from build123d import *

# Parameters (mm, degrees)
SKETCH133_W       = 5
SKETCH133_H       = 20
PAD080_DEPTH      = 20
SKETCH134_W       = 2.5
SKETCH134_H       = 15.6
POCKET028_DEPTH   = 18
CYLINDER086_R     = 6.5
CYLINDER086_DEPTH = 3
PAD081_DEPTH      = 2.5


with BuildPart() as part:
    # Sketch133 → Pad080 (new body)
    with BuildSketch(Plane.XY):
        with Locations((2.5, 0)):
            Rectangle(SKETCH133_W, SKETCH133_H)
    extrude(amount=-PAD080_DEPTH)

    # Sketch134 → Pocket028 (cut)
    with BuildSketch(Plane(origin=(2.5, 0, 0), x_dir=(1, 0, 0), z_dir=(0, 0, 1))):
        Rectangle(SKETCH134_W, SKETCH134_H)
    extrude(amount=-POCKET028_DEPTH, mode=Mode.SUBTRACT)

    # Cylinder086 → Cylinder086 (cut)
    with BuildSketch(Plane(origin=(3, 0, -11), x_dir=(0, 1, 0), z_dir=(1, 0, 0))):
        Circle(CYLINDER086_R)
    extrude(amount=CYLINDER086_DEPTH, mode=Mode.SUBTRACT)

    # Sketch135 → Pad081 (join, symmetric)
    with BuildSketch(Plane(origin=(0, 0, -2), x_dir=(1, 0, 0), z_dir=(0, -1, 0))):
        Polygon((-8, 0), (0, 0), (0, -16), align=None)
    extrude(amount=PAD081_DEPTH, both=True)


with BuildPart() as part_1:
    # Body118 placement: moved
    add(part.part.moved(Location((5, 0, 0))))


solid = part_1.part
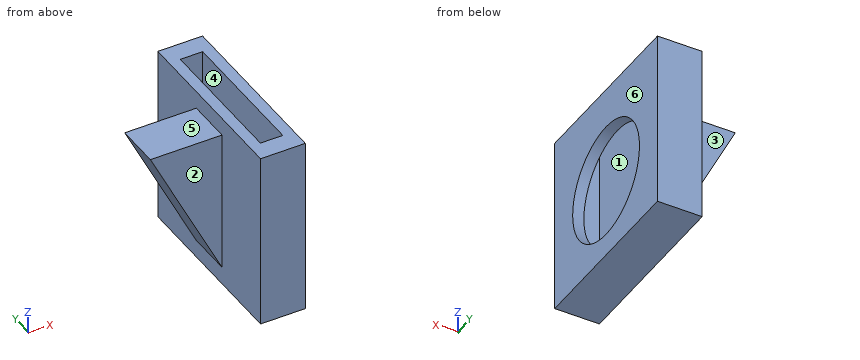
Can you work these out from the model? Positions are in its coordinate system, mm. Face numbers are marked on the shaded views. A direction names the side the tool comes from. Give positions to 0.01 mm unless a question says otherwise; leave off trailing zeros. Order: outer loops, then holes, each group sorted by start corner. A loop starts at its lowest first (then second) coordinate and runs counter-clockwise, first axis right, second up. Notation, with made-up numbers: M 19,66 L 61,66 A18 cw 61,84 Z; hole C -17.5,74.25 d8. An arc over 180 degrees is marked long. One line per question, with ' | ' between items.
Item 1: We'd pull the mould along X, two halves only. Please class the marked faces 4, 5 and 6: released by +X, released by -X, zero draft, split by the parting line, or undercut.
Answer block:
face 4: undercut | face 5: zero draft | face 6: released by +X
Item 2: Please list where these lines run through material, in increasing order: L1, parallel to Z at x = 9.1, y = 0; L2, parallel to X at y = -4, z = -1.5; L3, parallel to Y at x = 8, z = -6.25.
Answer block:
L1: z = -20 to -17.5, -4.5 to 0 | L2: x = 5 to 6.25, 8.75 to 10 | L3: y = -10 to -7.8, 7.8 to 10
Item 3: Suppose I cut it at C-C, the plane x = 9.25. Write out the boundary of the cut face in (y, z).
Answer block:
outline: M -10,-20 L 10,-20 L 10,0 L -10,0 Z; hole C 0,-11 d13
Item 4: Suppose I cut it at B-B, the plane z = -17. Write out the boundary of the cut face in (x, y).
Answer block:
outline: M 4.5,-2.5 L 5,-2.5 L 5,-10 L 10,-10 L 10,-2.5 L 8.75,-2.5 L 8.75,-7.8 L 6.25,-7.8 L 6.25,7.8 L 8.75,7.8 L 8.75,2.5 L 10,2.5 L 10,10 L 5,10 L 5,2.5 L 4.5,2.5 Z
Item 5: I'm going to push flat-ended pins straight in: pin 1 Ø4 at (x, y) = (0.5, 2) entering from -Z; pin 2 Ø6 at (y, z) = (4, -13) entering from -X; pin 3 Ø4 at (y, z) = (-0.5, -14.5) entering from -X. Where does each tip first touch, or does it pass through?
Answer block:
pin 1: stops at z = -13 | pin 2: stops at x = 1.2 | pin 3: stops at x = 2.25
Item 6: For the marked faces 1, 2 and 3, which set-ups out of +Z, -Z, +X, -X, +Y, -Y let a thin tool reach every point of the face, with its end or its side?
Answer block:
face 1: +Z | face 2: +Z, -Z, -X, -Y | face 3: +Z, -Z, -X, +Y
Item 7: Suppose I cut it at D-D, the plane z = -11. Write out the boundary of the cut face in (x, y).
Answer block:
outline: M 1.5,-2.5 L 5,-2.5 L 5,-10 L 10,-10 L 10,-6.5 L 8.75,-6.5 L 8.75,-7.8 L 6.25,-7.8 L 6.25,7.8 L 8.75,7.8 L 8.75,6.5 L 10,6.5 L 10,10 L 5,10 L 5,2.5 L 1.5,2.5 Z
Item 8: Suppose I cut it at A-A, the plane y = 0. Write out the boundary of the cut face in (x, z), then the cut area to 3 significant figures.
Answer block:
outline: M -3,-2 L 5,-18 L 5,-20 L 10,-20 L 10,-17.5 L 8.75,-17.5 L 8.75,-18 L 6.25,-18 L 6.25,0 L 5,0 L 5,-2 Z; M 8.75,-4.5 L 10,-4.5 L 10,0 L 8.75,0 Z | area: 103 mm2
